Source: CAD feature listing. Evaluate the final solid. Frame: model axes, mm. Give positions to 0.01 mm unless a question says otherwise; leave off trailing zeros. Order: outer loops, then holes, each group sorted by start corner. A loop starts at its lowest first (then second) coordinate and runs counter-clockwise, first axis right, second up. Notation, with made-up numbers: M -23.5,22.5 L 20.5,22.5 A13 ccw 20.5,47.5 Z; hole C 41,16.5 d8. An arc over 180 degrees is marked long. Use CSV: the item, a comma, the result in double quotes. Start each with the question number.
Item 1: Section query B-B on x = -7.25. Return loops of the section in (y, z), and give its area (3 significant figures).
Item 2: Section query A-A on y = 0.35. Return loops of the section in (x, z), and give its area (3 significant figures).
Item 3: Ray query, probe 1 along X at (y, z) = (0.6, -6.35); probe 2 along Z at (x, y) = (7.5, 1.2); probe 3 along Z at (x, y) = (8.5, 0.45). Return the intervals inside material, ascending. Write a range as from..to.
Item 4: First-contact query: pin 1 (2 mm diameter, centred on x = -7.62, z = -6.35, fed in from -Y). Flat tip, straight axial feed; report the tip coordinate or a pass-through.
Item 5: Pull-direction query (X, two-part tool) for faces 1 (the face through (-8.39, 0.62, -7.36)), 2 (the face through (10.16, 1, 0)), 3 (the face through (6.85, 0.62, -7.36)), 4 (the face through (-9.396, 0.616, 8.166)); classes: +X half, -X half, draft (parallel to the pull), parting line (faces both ways), or undercut.
from build123d import *

# Parameters (mm, degrees)
SKETCH1_R           = 1.27
BOSS_EXTRUDE1_DEPTH = 1.25


with BuildPart() as part:
    # Sketch1 → Boss-Extrude1 (new body)
    with BuildSketch(Plane(origin=(0, 0, 0), x_dir=(1, 0, 0), z_dir=(0, 1, 0))):
        with BuildLine():
            ThreePointArc((-7.62, -8.89), (-9.416051224, -8.146051224), (-10.16, -6.35))
            Line((-10.16, -6.35), (-10.16, 6.35))
            ThreePointArc((-10.16, 6.35), (-9.416051224, 8.146051224), (-7.62, 8.89))
            Line((-7.62, 8.89), (7.62, 8.89))
            ThreePointArc((7.62, 8.89), (9.416051224, 8.146051224), (10.16, 6.35))
            Line((10.16, 6.35), (10.16, -6.35))
            ThreePointArc((10.16, -6.35), (9.416051224, -8.146051224), (7.62, -8.89))
            Line((7.62, -8.89), (-7.62, -8.89))
        make_face()
        with Locations(Location((7.62, 6.35, 0), (0, 0, 270))):
            Circle(SKETCH1_R, mode=Mode.SUBTRACT)
        with Locations(Location((-7.62, 6.35, 0), (0, 0, 270))):
            Circle(SKETCH1_R, mode=Mode.SUBTRACT)
    extrude(amount=BOSS_EXTRUDE1_DEPTH)


solid = part.part
Verdict:
1,outline,"M 0,-8.89 L 1.25,-8.89 L 1.25,-7.56 L 0,-7.56 Z; M 0,-5.14 L 1.25,-5.14 L 1.25,8.89 L 0,8.89 Z"
1,area,"19.2 mm2"
2,outline,"M -10.16,-6.35 A2.54 ccw -7.62,-8.89 L 7.62,-8.89 A2.54 ccw 10.16,-6.35 L 10.16,6.35 A2.54 ccw 7.62,8.89 L -7.62,8.89 A2.54 ccw -10.16,6.35 Z; hole C -7.62,-6.35 d2.54; hole C 7.62,-6.35 d2.54"
2,area,"346 mm2"
3,probe 1,"-10.16..-8.89, -6.35..6.35, 8.89..10.16"
3,probe 2,"-8.89..-7.61, -5.09..8.89"
3,probe 3,"-8.73..-7.27, -5.43..8.73"
4,pin 1,"through"
5,face 1,"undercut"
5,face 2,"+X half"
5,face 3,"undercut"
5,face 4,"-X half"
